The listing builds one solid part. Answer for the finished solid, in the listing's coordinates (mm). Face numbers are marked on the shaded views. Give positions to 0.01 mm unless a question says otherwise; leave off trailing zeros. Write each loop counter-clockwise with the first axis right and the second up, starting at its lowest first coordinate (ties: lowest second). Pieces come first, ordered by that corner, then holes. Notation, with made-up numbers: (66, 33) - (118, 33) arc R16 cw to (118, 39) - close; hole circle Ø3 at (-24, 77). An arc over 180 degrees is marked (long way). Use a Markdown table: item, result. Add a question column.
from build123d import *

# Parameters (mm, degrees)
SKETCH1_W           = 200
SKETCH1_H           = 30
BOSS_EXTRUDE1_DEPTH = 30
FILLET1_R           = 10
CUT_EXTRUDE1_DEPTH  = 30
SKETCH3_W           = 7.5
SKETCH3_H           = 30
CUT_EXTRUDE2_DEPTH  = 26
SKETCH4_W           = 7.5
SKETCH4_H           = 30
CUT_EXTRUDE3_DEPTH  = 26
SKETCH5_R           = 10
CUT_EXTRUDE4_DEPTH  = 45
SCALE1_SCALE        = 4


with BuildPart() as part:
    # Sketch1 → Boss-Extrude1 (new body)
    with BuildSketch(Plane.XY):
        with Locations((46.259717806, -4.797058824)):
            Rectangle(SKETCH1_W, SKETCH1_H)
    extrude(amount=BOSS_EXTRUDE1_DEPTH)

    # Fillet1
    fillet1_edges = [part.edges().sort_by_distance(p)[0] for p in [
        (-53.740282194, 10.202941176, 15),
        (146.259717806, 10.202941176, 15),
        (146.259717806, -19.797058824, 15),
        (-53.740282194, -19.797058824, 15),
    ]]
    fillet(fillet1_edges, radius=FILLET1_R)

    # Sketch2 → Cut-Extrude1 (cut)
    with BuildSketch(Plane.XY.offset(30)):
        with BuildLine():
            Line((-27.901084514, 10.202941176), (70.420520136, 10.202941176))
            ThreePointArc((70.420520136, 10.202941176), (21.259717811, 5.202941178), (-27.901084514, 10.202941176))
        make_face()
        with BuildLine():
            Line((-27.901084524, -19.797058824), (70.420520136, -19.797058824))
            ThreePointArc((70.420520136, -19.797058824), (21.259717806, -14.798405243), (-27.901084524, -19.797058824))
        make_face()
    extrude(amount=-CUT_EXTRUDE1_DEPTH, mode=Mode.SUBTRACT)

    # Sketch3 → Cut-Extrude2 (cut)
    with BuildSketch(Plane(origin=(146.259717806, 0, 0), x_dir=(0, 0, -1), z_dir=(1, 0, 0))):
        with Locations((-3.75, -4.797058824)):
            Rectangle(SKETCH3_W, SKETCH3_H)
        with Locations((-26.25, -4.797058824)):
            Rectangle(SKETCH3_W, SKETCH3_H)
    extrude(amount=-CUT_EXTRUDE2_DEPTH, mode=Mode.SUBTRACT)

    # Sketch4 → Cut-Extrude3 (cut)
    with BuildSketch(Plane.ZY.offset(53.740282194)):
        with Locations((26.25, -4.797058824)):
            Rectangle(SKETCH4_W, SKETCH4_H)
        with Locations((3.75, -4.797058824)):
            Rectangle(SKETCH4_W, SKETCH4_H)
    extrude(amount=-CUT_EXTRUDE3_DEPTH, mode=Mode.SUBTRACT)

    # Sketch5 → Cut-Extrude4 (cut)
    with BuildSketch(Plane.XY.offset(30)):
        with Locations((-39.286224807, -4.797058824)):
            Circle(SKETCH5_R)
        with Locations((133.184735123, -4.797058824)):
            Circle(SKETCH5_R)
    extrude(amount=-CUT_EXTRUDE4_DEPTH, mode=Mode.SUBTRACT)


with BuildPart() as part_1:
    # Scale1: scaled about (50.111608126, -4.79729109, 15)
    add(part.part.scale(SCALE1_SCALE).moved(Location((-150.334824378, 14.39187327, -45))))


solid = part_1.part
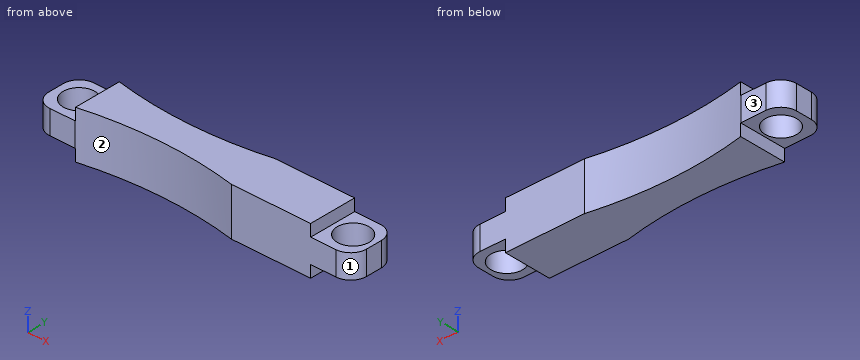
1. For a pull along X with two mould halves and no side action, classify the marked faces 1, 2 and 3 as released by +X, released by -X, zero draft, split by the parting line, or undercut.
2. Consider L1, parallel to X at y = -34, z = 35; L2, parallel to X at y = -6, z = 2; L3, parallel to X at y = 13, z = 45.5. Determine where each line is inside the solid, lowest interval first. Write a range as [from, to].
3. The part is cut by section C-C (x = -174.5). Give the vertices of the cut face in (y, z).
4. The part is cut by section B-B (z = -6.5). Give the vertices of the cut face in (x, y), and give its area (3 significant figures).
5. Given P1, Ø15, axis at y = 17.5, z = -25.5, coming from the -X side; P2, Ø3, axis at x = -199.5, z = 25, coming from the +Y side; P3, Ø3, axis at y = 25.5, z = 40.5, coming from the -X side, each flat-ended and moving along its own axis, determine where each tip first touches the part or whether it passes through.
6. The part is cut by section A-A (y = 22.5). Give the vertices of the cut face in (x, z), and give its area (3 significant figures).
Check values:
| question | item | result |
|---|---|---|
| 1 | face 1 | released by +X |
| 1 | face 2 | undercut |
| 1 | face 3 | zero draft |
| 2 | L1 | x = [-364.22, -334.81], [-280.15, 355.07], [409.74, 433.63] |
| 2 | L2 | x = [-365.3, -347.46], [-267.5, 342.42], [422.39, 434.7] |
| 2 | L3 | x = [-261.3, 330.7] |
| 3 | outline | (-50.92, -45) - (41.33, -45) - (41.33, 75) - (-50.92, 75) - close |
| 4 | outline | (-365.3, -24.8) arc R40 ccw to (-325.3, -64.8) - (-261.94, -64.8) arc R976.97 cw to (131.35, -64.8) - (394.7, -64.8) arc R40 ccw to (434.7, -24.8) - (434.7, 15.2) arc R40 ccw to (394.7, 55.2) - (131.35, 55.2) arc R976.71 cw to (-261.94, 55.2) - (-325.3, 55.2) arc R40 ccw to (-365.3, 15.2) - close; hole circle Ø80 at (-307.48, -4.8); hole circle Ø80 at (382.4, -4.8) |
| 4 | area | 74,100 mm2 |
| 5 | P1 | stops at x = -261.3 |
| 5 | P2 | stops at y = 44.68 |
| 5 | P3 | stops at x = -364.32 |
| 6 | outline | (-364.62, -15) - (-336.72, -15) - (-336.72, 45) - (-364.62, 45) - close; (-278.24, -15) - (-261.3, -15) - (-261.3, -45) - (330.7, -45) - (330.7, -15) - (353.17, -15) - (353.17, 45) - (330.7, 45) - (330.7, 75) - (-261.3, 75) - (-261.3, 45) - (-278.24, 45) - close; (411.64, -15) - (434.03, -15) - (434.03, 45) - (411.64, 45) - close |
| 6 | area | 76,400 mm2 |
